The listing builds one solid part. Answer for the finished solid, in the listing's coordinates (mm). A direction names the side the tool comes from. Coordinates: 2 decimals unless noted, no trailing zeros. Write each loop counter-clockwise with the first axis right and the second up, starting at its lowest first coordinate (ties: lowest second). Pieces come first, ordered by that corner, then holes. Notation, with made-up numbers: M 65.25,-10.75 L 89.25,-10.75 A24 cw 89.25,23.25 Z; hole C 24,25 d6. An arc over 180 degrees is marked long. Put each result on its own line as item: value. Start each with the question number.
```python
from build123d import *

# Parameters (mm, degrees)
SKETCH006_R      = 15.9
SKETCH006_R_2    = 14
EXTRUDE006_DEPTH = 3
SKETCH005_R      = 2.3
EXTRUDE005_DEPTH = 12
SKETCH004_R      = 25
SKETCH004_R_2    = 14
EXTRUDE004_DEPTH = 4


with BuildPart() as extrude006:
    # Sketch006 → Extrude006 (new body)
    with BuildSketch(Plane.XY):
        Circle(SKETCH006_R)
        Circle(SKETCH006_R_2, mode=Mode.SUBTRACT)
    extrude(amount=EXTRUDE006_DEPTH)


with BuildPart() as extrude006_1:
    # Extrude006 placement: moved
    add(extrude006.part.moved(Location((0, 0, 4))))


with BuildPart() as extrude005:
    # Sketch005 → Extrude005 (new body)
    with BuildSketch(Plane.XY):
        with Locations((-20, 0)):
            Circle(SKETCH005_R)
        with Locations((0, -20)):
            Circle(SKETCH005_R)
        with Locations((20, 0)):
            Circle(SKETCH005_R)
        with Locations((0, 20)):
            Circle(SKETCH005_R)
    extrude(amount=EXTRUDE005_DEPTH)


with BuildPart() as fusion:
    # Sketch004 → Extrude004 (new body)
    with BuildSketch(Plane.XY):
        Circle(SKETCH004_R)
        Circle(SKETCH004_R_2, mode=Mode.SUBTRACT)
    extrude(amount=EXTRUDE004_DEPTH)

    # Cut: cut Extrude005
    add(extrude005.part, mode=Mode.SUBTRACT)

    # Fusion: union Extrude006
    add(extrude006_1.part)


solid = fusion.part
```
1) Straight lines are drawn through the part: probe 1 along Y at (x, z) = (0, 1.5); probe 2 along Z at (x, y) = (0.5, -16.5); probe 3 along X at (y, z) = (20, 2). For each, find the intervals that lie inside material, in ascending order.
2) A cutting plane is placed at A-A on x = 20. Write down the section's boundary in (y, z).
3) Given pin 1 Ø1 at (x, z) = (5, 6) entering from -Y; pin 2 Ø1.5 at (y, z) = (7, 3) entering from -X; pin 3 Ø1 at (x, y) = (13, 17.5) entering from +Z, each flat-ended and moving along its own axis, determine where each tip first touches the part or whether it passes through.
4) Determine the mould class of faces 3 (the face through (11, -11, 0)), 4 (the face through (-0.499, -22.245, 1.972)), 5 (the face through (23.846, 7.509, 1.972)) for opening direction Y: +Y half, -Y half, draft (parallel to the pull), parting line (faces both ways), or undercut.
5) A cutting plane is placed at C-C on x = 0. Write down the section's boundary in (y, z), then the cut area to 3 significant figures.
6) For faces 1 (the face through (-3.45, -15.52, 5.48)), 2 (the face through (12.932, -5.362, 3.451)), determine the directions among +Z, -Z, +X, -X, +Y, -Y from which every point of the face is accessible in a straight line to the end or side of a thin tool.
Answers follow:
1. probe 1: y = -25 to -22.3, -17.7 to -14, 14 to 17.7, 22.3 to 25
1. probe 2: z = 0 to 4
1. probe 3: x = -15 to -2.3, 2.3 to 15
2. outline: M -15,0 L -2.3,0 L -2.3,4 L -15,4 Z; M 2.3,0 L 15,0 L 15,4 L 2.3,4 Z
3. pin 1: stops at y = -15.25
3. pin 2: stops at x = -24.21
3. pin 3: stops at z = 4
4. face 3: draft
4. face 4: undercut
4. face 5: parting line
5. outline: M -25,0 L -22.3,0 L -22.3,4 L -25,4 Z; M -17.7,0 L -14,0 L -14,7 L -15.9,7 L -15.9,4 L -17.7,4 Z; M 14,0 L 17.7,0 L 17.7,4 L 15.9,4 L 15.9,7 L 14,7 Z; M 22.3,0 L 25,0 L 25,4 L 22.3,4 Z
5. area: 62.6 mm²
6. face 1: +Z
6. face 2: +Z, -Z
